```python
from build123d import *

# Parameters (mm, degrees)
ESQUISSE1_W             = 0.5
ESQUISSE1_H             = 56.8
EXTRUSION1_DEPTH        = 13.5
EXTRUSION1_2_DEPTH      = 13.5
ESQUISSE1_W_2           = 19.9
ESQUISSE1_H_2           = 0.5
EXTRUSION1_3_DEPTH      = 13.5
EXTRUSION1_4_DEPTH      = 13.5
ESQUISSE2_W             = 19.9
ESQUISSE2_H             = 58
EXTRUSION2_DEPTH        = 0.5
ENL_V_MAT_EXTRU_1_DEPTH = 10.5
ESQUISSE4_W             = 0.5
ESQUISSE4_H             = 1
EXTRUSION3_DEPTH        = 2


with BuildPart() as part:
    # Esquisse1 → Extrusion1 (new body)
    with BuildSketch(Plane.XY):
        with Locations((91.99228109, 2.086823856)):
            Rectangle(ESQUISSE1_W, ESQUISSE1_H)
    extrude(amount=EXTRUSION1_DEPTH)



with BuildPart() as body_2:
    # Esquisse1 → Extrusion1 2 (new body)
    with BuildSketch(Plane.XY):
        with Locations((111.39228109, 2.086823856)):
            Rectangle(ESQUISSE1_W, ESQUISSE1_H)
    extrude(amount=EXTRUSION1_2_DEPTH)


with BuildPart() as body_3:
    # Esquisse1 → Extrusion1 3 (new body)
    with BuildSketch(Plane.XY):
        with Locations((101.69228109, 30.836823856)):
            Rectangle(ESQUISSE1_W_2, ESQUISSE1_H_2)
    extrude(amount=EXTRUSION1_3_DEPTH)


with BuildPart() as body_4:
    # Esquisse1 → Extrusion1 4 (new body)
    with BuildSketch(Plane.XY):
        with Locations((101.69228109, -26.663176144)):
            Rectangle(ESQUISSE1_W_2, ESQUISSE1_H_2)
    extrude(amount=EXTRUSION1_4_DEPTH)


with BuildPart() as part_1:
    add(part.part)

    add(body_2.part)  # Extrusion2 merges body 2

    add(body_3.part)  # Extrusion2 merges body 3

    add(body_4.part)  # Extrusion2 merges body 4
    # Esquisse2 → Extrusion2 (add)
    with BuildSketch(Plane.XY.offset(13.5)):
        with Locations((101.69228109, 2.086823856)):
            Rectangle(ESQUISSE2_W, ESQUISSE2_H)
    extrude(amount=EXTRUSION2_DEPTH)

    # Esquisse3 → Enlèv. mat.-Extru.1 (cut)
    with BuildSketch(Plane(origin=(111.64228109, 0, 0), x_dir=(0, 0, -1), z_dir=(1, 0, 0))):
        with BuildLine():
            Line((0, 22.321054975), (0, 18.821054975))
            Line((0, 18.821054975), (-3.3, 18.821054975))
            ThreePointArc((-3.3, 18.821054975), (-5.05, 20.571054975), (-3.3, 22.321054975))
            Line((-3.3, 22.321054975), (0, 22.321054975))
        make_face()
        with BuildLine():
            Line((0, 3.321054975), (0, -0.178945025))
            Line((0, -0.178945025), (-3.3, -0.178945025))
            ThreePointArc((-3.3, -0.178945025), (-5.05, 1.571054975), (-3.3, 3.321054975))
            Line((-3.3, 3.321054975), (0, 3.321054975))
        make_face()
        with BuildLine():
            Line((0, -15.678945025), (0, -19.178945025))
            Line((0, -19.178945025), (-3.3, -19.178945025))
            ThreePointArc((-3.3, -19.178945025), (-5.05, -17.428945025), (-3.3, -15.678945025))
            Line((-3.3, -15.678945025), (0, -15.678945025))
        make_face()
    extrude(amount=-ENL_V_MAT_EXTRU_1_DEPTH, mode=Mode.SUBTRACT)

    # Esquisse4 → Extrusion3 (add)
    with BuildSketch(Plane(origin=(0, 0, 0), x_dir=(-1, 0, 0), z_dir=(0, 0, -1))):
        with Locations((-111.39228109, 26.536823856)):
            Rectangle(ESQUISSE4_W, ESQUISSE4_H)
        with Locations((-91.99228109, 26.536823856)):
            Rectangle(ESQUISSE4_W, ESQUISSE4_H)
        with Locations((-111.39228109, -22.363176144)):
            Rectangle(ESQUISSE4_W, ESQUISSE4_H)
        with Locations((-91.99228109, -22.363176144)):
            Rectangle(ESQUISSE4_W, ESQUISSE4_H)
    extrude(amount=EXTRUSION3_DEPTH)


solid = part_1.part
```
Geometry check sheet. Reference: the model listing, model coordinates, mm. A direction names the side the tool comes from. Give positions to 0.01 mm unless a question says otherwise; leave off trailing zeros. Order: outer loops, then holes, each group sorted by start corner. A loop starts at its lowest first (then second) coordinate and runs counter-clockwise, first axis right, second up.
1. Section check A-A, the plane z = 11. Enter the section's corners in (x, y).
2. Section check B-B, the plane z = 0.75. Enter the section's corners in (x, y).
3. Gauge pin test, flat ends, axial feed: pin 1 Ø0.6 at (x, z) = (92, -1.5) entering from +Y; pin 2 Ø10 at (x, y) = (102.5, -3) entering from -Z; pin 3 Ø0.6 at (x, y) = (99, 31) entering from -Z. Record the tip position at first contact, or that the pin passes through.
4. Access from +Z, -Z, +X, -X, +Y, -Y to the whole of each face (thin tool, end or side, straight path). Record for faces 1 (the face through (111.4, 20.53, 5.05)), 2 (the face through (111.642, 2, 8)), 3 (the face through (102, 31.087, 7)), 4 (the face through (111.142, 2, 7)), 5 (the face through (102, 30.587, 7)).
5. Thickness scan on L1, parallel to X at y = -11.5, z = 8.25; L2, parallel to Y at x = 97.75, z = 3.5; L3, parallel to Z at x = 109, y = -19. Record the ranges inside material, lowest first.
6. Section check D-D, the plane y = 10.5. Enter the section's corners in (x, z).
7. Release check for a two-part mould opening along X. For faces 6 (the face through (102, 2, 14)), 7 (the face through (91.742, 2, 6)), 8 (the face through (92.242, 2, 6)) record: pulls with the +X half, pulls with the -X half, needs draft (parallel to the pull), parting line crosses it, or undercut.
8. Section check C-C, the plane x = 97. Enter the section's corners in (y, z).
Values follow:
1. outline: (91.74, -26.91) - (111.64, -26.91) - (111.64, -26.41) - (91.74, -26.41) - close; (91.74, -26.31) - (92.24, -26.31) - (92.24, 30.49) - (91.74, 30.49) - close; (91.74, 30.59) - (111.64, 30.59) - (111.64, 31.09) - (91.74, 31.09) - close; (111.14, -26.31) - (111.64, -26.31) - (111.64, 30.49) - (111.14, 30.49) - close
2. outline: (91.74, -26.91) - (111.64, -26.91) - (111.64, -26.41) - (91.74, -26.41) - close; (91.74, -26.31) - (92.24, -26.31) - (92.24, 30.49) - (91.74, 30.49) - close; (91.74, 30.59) - (111.64, 30.59) - (111.64, 31.09) - (91.74, 31.09) - close; (111.14, -26.31) - (111.64, -26.31) - (111.64, -19.18) - (111.14, -19.18) - close; (111.14, -15.68) - (111.64, -15.68) - (111.64, -0.18) - (111.14, -0.18) - close; (111.14, 3.32) - (111.64, 3.32) - (111.64, 18.82) - (111.14, 18.82) - close; (111.14, 22.32) - (111.64, 22.32) - (111.64, 30.49) - (111.14, 30.49) - close
3. pin 1: stops at y = 27.04
3. pin 2: stops at z = 13.5
3. pin 3: stops at z = 0
4. face 1: -Z, +X
4. face 2: +Z, -Z, +X, +Y, -Y
4. face 3: +Z, -Z, +X, -X, +Y
4. face 4: -Z
4. face 5: -Z, +X, -X
5. L1: x = 91.74 to 92.24, 111.14 to 111.64
5. L2: y = -26.91 to -26.41, 30.59 to 31.09
5. L3: z = 13.5 to 14
6. outline: (91.74, 0) - (92.24, 0) - (92.24, 13.5) - (111.14, 13.5) - (111.14, 0) - (111.64, 0) - (111.64, 14) - (91.74, 14) - close
7. face 6: needs draft
7. face 7: pulls with the -X half
7. face 8: undercut
8. outline: (-26.91, 0) - (-26.41, 0) - (-26.41, 13.5) - (30.59, 13.5) - (30.59, 0) - (31.09, 0) - (31.09, 14) - (-26.91, 14) - close
